For this review, use the dimensioned drawing (mm, ordinates from the lowest corner) and the shaded views. A direction names the side the tool comes from. Give positions to 0.01 mm unless a question says otherwise; leave off trailing zeros. Write each loop counter-clockwise with the first axis right and the second up, starting at its lowest first coordinate (ties: lowest second). Pieces come first, ordered by that corner, then holes.
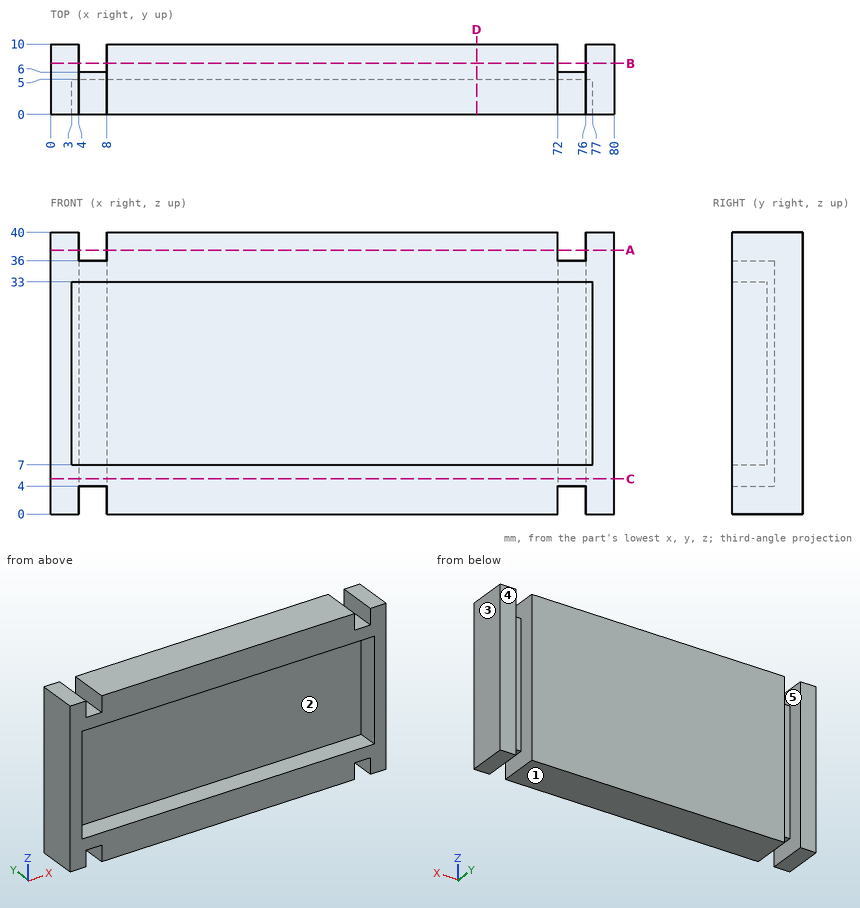
(1) We need section A-A (z = 37.5). Write out the cut boundary in (x, y), and give its area (3 significant figures).
(2) The part is to be moulded in two halves that separate along X. For the marked faces 3, 4 and 5, say which applies: +X half, -X half, draft (parallel to the pull), parting line (faces both ways), or undercut.
(3) Clearance check with flat-ended pins moving along their axes: pin 1 Ø8 at (x, z) = (64.5, 23.5) entering from -Y; pin 2 Ø3 at (x, z) = (6, 12.5) entering from +Y. State where each tip first meets the part, or that it passes through.
(4) Tool access review of the marked faces 1 and 2: name each direction out of +Z, -Z, +X, -X, +Y, -Y from which nothing blocks a thin tool from reaching the whole face with its end or side.
(5) We need section D-D (x = 60.5). Write out the cut boundary in (y, z), and give its area (3 significant figures).
(6) We need section B-B (y = 7.25). Write out the cut boundary in (x, z), and give its area (3 significant figures).
(7) For L1, parallel to X at y = 3.5, z = 3; L2, parallel to X at y = 4, z = 17.5; L3, parallel to Z at x = 49.5, y = 2.25, list the stretches that pass through material, from the lowest coordinate up.
(8) We need section C-C (z = 5). Write out the cut boundary in (x, y), and give its area (3 significant figures).
The answers:
1. outline: (0, 0) - (4, 0) - (4, 10) - (0, 10) - close; (8, 0) - (72, 0) - (72, 10) - (8, 10) - close; (76, 0) - (80, 0) - (80, 10) - (76, 10) - close
1. area: 720 mm2
2. face 3: +X half
2. face 4: draft
2. face 5: undercut
3. pin 1: stops at y = 5
3. pin 2: stops at y = 6
4. face 1: -Z, +X, -X, +Y, -Y
4. face 2: -Y
5. outline: (0, 0) - (10, 0) - (10, 40) - (0, 40) - (0, 33) - (5, 33) - (5, 7) - (0, 7) - close
5. area: 270 mm2
6. outline: (0, 0) - (4, 0) - (4, 40) - (0, 40) - close; (8, 0) - (72, 0) - (72, 40) - (8, 40) - close; (76, 0) - (80, 0) - (80, 40) - (76, 40) - close
6. area: 2,880 mm2
7. L1: x = 0 to 4, 8 to 72, 76 to 80
7. L2: x = 0 to 3, 77 to 80
7. L3: z = 0 to 7, 33 to 40
8. outline: (0, 0) - (80, 0) - (80, 10) - (76, 10) - (76, 6) - (72, 6) - (72, 10) - (8, 10) - (8, 6) - (4, 6) - (4, 10) - (0, 10) - close
8. area: 768 mm2
